For this review, use the dimensioned drawing (mm, ordinates from the lowest corner) and the shaded views. A direction names the side the tool comes from. Coordinates: 2 decimals unless noted, no trailing zeros. Write each loop counter-clockwise with the first axis right and the second up, starting at its lowest first coordinate (ties: lowest second). Pieces come first, ordered by that corner, then holes. Notation, with made-up numbers: (27.25, -13.75) - (54.25, -13.75) arc R20 ccw to (54.25, -3.75) - close; hole circle Ø11 at (-31.5, 63). An arc over 180 degrees is marked (long way). Use one line per item in the form item = value. Start each with the question number.
1) Mouldability with a two-part tool opening along X and no side actions: class the marked faces 1, 2, 3 and 4 as pulls with the +X half, pulls with the -X half, needs draft (parallel to the pull), parting line crosses it, or undercut.
2) Tool access review of the marked faces 5 and 6: name each direction out of +Z, -Z, +X, -X, +Y, -Y from which nothing blocks a thin tool from reaching the whole face with its end or side.
3) Insertion check: P1, Ø3, axis at x = 17.5, z = 16, coming from the -Y side. The pin has a flat end and moves straight along its axis. Give the tip position at first contact, or say it passes through.
4) For L1, parallel to X at y = 10.5, z = 13.25; L2, parallel to X at y = 36.5, z = 6; L3, parallel to Y at x = 39.1, z = 4, list the stretches that pass through material, from the lowest coordinate up. Write a range as from..to.
5) We need section B-B (z = 18). Give the boundary of the cut face in (x, y), plus the area to 3 significant figures.
6) We need section A-A (x = 27). Give the boundary of the cut face in (y, z), plus the area to 3 significant figures.
7) We need section C-C (y = 35). Give the boundary of the cut face in (x, z).
8) We need section D-D (x = 15). Give the boundary of the cut face in (y, z).
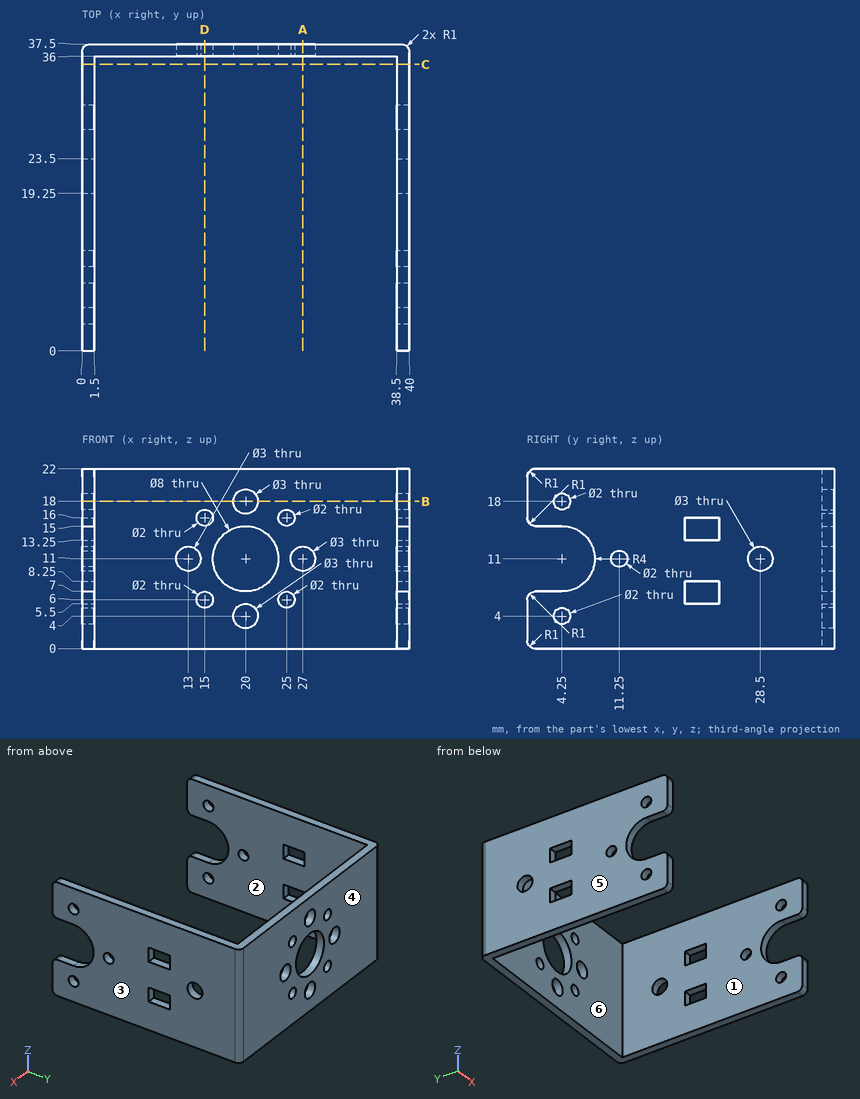
Determined:
q1.face_1 = undercut
q1.face_2 = undercut
q1.face_3 = pulls with the +X half
q1.face_4 = needs draft
q2.face_5 = +Z, -Z, -X, +Y, -Y
q2.face_6 = +Z, -Z, -Y
q3.P1 = 36
q4.L1 = 0..1.5, 38.5..40
q4.L2 = 0..14, 16..24, 26..40
q4.L3 = 0..3.25, 5.25..37.49
q5.outline = (0, 0) - (1.5, 0) - (1.5, 3.25) - (0, 3.25) - close; (0, 5.25) - (1.5, 5.25) - (1.5, 36) - (18.5, 36) - (18.5, 37.5) - (1, 37.5) arc R1 ccw to (0, 36.5) - close; (21.5, 36) - (38.5, 36) - (38.5, 5.25) - (40, 5.25) - (40, 36.5) arc R1 ccw to (39, 37.5) - (21.5, 37.5) - close; (38.5, 0) - (40, 0) - (40, 3.25) - (38.5, 3.25) - close
q5.area = 157 mm²
q6.outline = (36, 0) - (37.5, 0) - (37.5, 9.5) - (36, 9.5) - close; (36, 12.5) - (37.5, 12.5) - (37.5, 22) - (36, 22) - close
q6.area = 28.5 mm²
q7.outline = (0, 0) - (1.5, 0) - (1.5, 22) - (0, 22) - close; (38.5, 0) - (40, 0) - (40, 22) - (38.5, 22) - close
q8.outline = (36, 0) - (37.5, 0) - (37.5, 5) - (36, 5) - close; (36, 7) - (37.5, 7) - (37.5, 15) - (36, 15) - close; (36, 17) - (37.5, 17) - (37.5, 22) - (36, 22) - close
